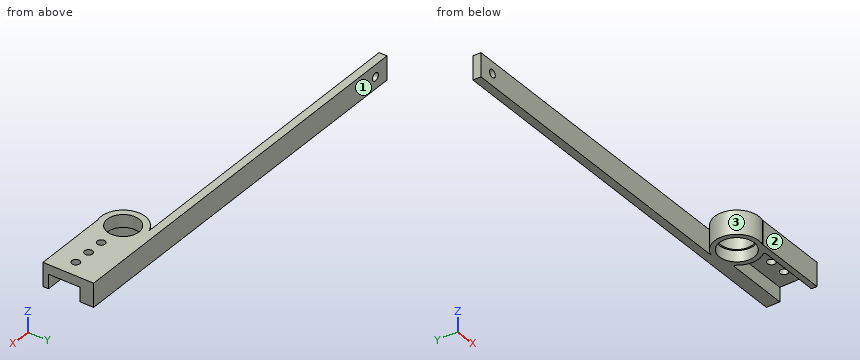
```python
from build123d import *

# Parameters (mm, degrees)
SKETCH_1_W          = 40
SKETCH_1_H          = 20
EXTRUDE_1_DEPTH     = 6
SKETCH_2_R          = 2.5
CUT_EXTRUDE_1_DEPTH = 24.151673806
EXTRUDE_START       = -15
EXTRUDE_2_OUTLINE_R = 11
EXTRUDE_2_DEPTH     = 15
EXTRUDE_START_2     = -8
SKETCH_5_R          = 11
SKETCH_5_R_2        = 10
EXTRUDE_3_DEPTH     = 8
SKETCH_8_W          = 15
SKETCH_8_H          = 5
EXTRUDE_4_DEPTH     = 500
SKETCH_9_W          = 4.037306924
SKETCH_9_H          = 3.364422437
EXTRUDE_5_DEPTH     = 15
SKETCH_11_W         = 261.320344598
SKETCH_11_H         = 37.265148186
CUT_EXTRUDE_2_DEPTH = 482.183177179
SKETCH_12_R         = 2.5
CUT_EXTRUDE_3_DEPTH = 237.730557242


# Read off the part's stored shape, not the designer's step: 凸台-拉伸2
with BuildPart() as part:
    # 草图1 → 凸台-拉伸1 (new body)
    with BuildSketch(Plane.XY):
        Rectangle(SKETCH_1_W, SKETCH_1_H)
    extrude(amount=EXTRUDE_1_DEPTH)

    # 草图2 → 切除-拉伸1 (cut, through all)
    with BuildSketch(Plane.XY.offset(6)):
        with Locations((10, 0)):
            Circle(SKETCH_2_R)
        with Locations((-1, 0)):
            Circle(SKETCH_2_R)
        with Locations((-12, 0)):
            Circle(SKETCH_2_R)
    extrude(amount=-CUT_EXTRUDE_1_DEPTH, mode=Mode.SUBTRACT)

    # 凸台-拉伸2 outline → 凸台-拉伸2 (add)
    with BuildSketch(Plane.XY.offset(6).offset(EXTRUDE_START)):
        with BuildLine():
            Line((20, 10), (20, 13.5))
            Line((20, 13.5), (-26.893967141, 13.5))
            Line((-26.893967141, 13.5), (-26.893967141, 13.384337644))
            ThreePointArc((-26.893967141, 13.384337644), (-45, 0), (-26.893967141, -13.384337644))
            Line((-26.893967141, -13.384337644), (-26.893967141, -13.5))
            Line((-26.893967141, -13.5), (20, -13.5))
            Line((20, -13.5), (20, -10))
            Line((20, -10), (-20, -10))
            Line((-20, -10), (-20, -8.660254038))
            ThreePointArc((-20, -8.660254038), (-17, 0), (-20, 8.660254038))
            Line((-20, 8.660254038), (-20, 10))
            Line((-20, 10), (20, 10))
        make_face()
        with Locations((-31, 0)):
            Circle(EXTRUDE_2_OUTLINE_R, mode=Mode.SUBTRACT)
    extrude(amount=EXTRUDE_2_DEPTH)

    # 草图5 → 凸台-拉伸3 (add)
    with BuildSketch(Plane.XY.offset(6).offset(EXTRUDE_START_2)):
        with Locations((-31, 0)):
            Circle(SKETCH_5_R)
        with Locations((-31, 0)):
            Circle(SKETCH_5_R_2, mode=Mode.SUBTRACT)
    extrude(amount=EXTRUDE_3_DEPTH)

    # 草图8 → 凸台-拉伸4 (add)
    with BuildSketch(Plane(origin=(20, 0, 0), x_dir=(0, 0, -1), z_dir=(1, 0, 0))):
        with Locations((1.5, 16)):
            Rectangle(SKETCH_8_W, SKETCH_8_H)
    extrude(amount=-EXTRUDE_4_DEPTH)

    # 草图9 → 凸台-拉伸5 (add, through all)
    with BuildSketch(Plane(origin=(0, 0, -9), x_dir=(-1, 0, 0), z_dir=(0, 0, -1))):
        with Locations((26.475334378, 14.151164675)):
            Rectangle(SKETCH_9_W, SKETCH_9_H)
    extrude(amount=-EXTRUDE_5_DEPTH)

    # 草图11 → 切除-拉伸2 (cut, through all)
    with BuildSketch(Plane(origin=(0, 18.5, 0), x_dir=(1, 0, 0), z_dir=(0, 1, 0))):
        with Locations((-364.976425965, 6.732710128)):
            Rectangle(SKETCH_11_W, SKETCH_11_H)
    extrude(amount=-CUT_EXTRUDE_2_DEPTH, mode=Mode.SUBTRACT)

    # 草图12 → 切除-拉伸3 (cut, through all)
    with BuildSketch(Plane(origin=(0, 18.5, 0), x_dir=(1, 0, 0), z_dir=(0, 1, 0))):
        with Locations(Location((-224.316253666, 1.5, 0), (0, 0, 270))):
            Circle(SKETCH_12_R)
    extrude(amount=-CUT_EXTRUDE_3_DEPTH, mode=Mode.SUBTRACT)


solid = part.part
```
For this review, take the finished solid that the model builds, in its own axes (mm). Face numbers are marked on the shaded views. Give positions to 0.01 mm unless a question says otherwise; leave off trailing zeros. Write each loop counter-clockwise with the first axis right and the second up, starting at its lowest first coordinate (ties: lowest second). Pieces come first, ordered by that corner, then holes.
Item 1: Take a section at D-D (y = 5). Give the boundary of the cut face in (x, z), and give its area (3 significant figures).
Item 2: Take a section at C-C (x = -146). Give the boundary of the cut face in (y, z).
Item 3: Take a section at A-A (x = -12). Give the boundary of the cut face in (y, z), and give its area (3 significant figures).
Item 4: The part is to be moulded in two halves that separate along Y. For the marked faces 1, 2 and 3, say which applies: +Y half, -Y half, draft (parallel to the pull), parting line (faces both ways), or undercut.
Item 5: Take a section at B-B (y = -5.5). Give the boundary of the cut face in (x, z).
Item 6: Insertion check: P1, Ø6.5, axis at x = 10, y = 0, coming from the -Z side; P2, Ø7.5, axis at x = -8.5, z = -2.5, coming from the -Y side; P3, Ø4, axis at x = -66, z = 0, coming from the -Y side. Each pin has a flat end and moves straight along its axis. Give the tip position at first contact, or say it passes through.
Item 7: Wall thickness on probe 1 along Y at (x, z) = (-31, -5.25); probe 2 along X at (y, z) = (-1, 1); probe 3 along Y at (x, z) = (-1, 4.3): over which ranges is each line inside the solid? List them lowest first.
Established:
1. outline: (-44.08, -9) - (-40.8, -9) - (-40.8, -2) - (-39.66, -2) - (-39.66, 6) - (-44.08, 6) - close; (-22.34, -2) - (-21.2, -2) - (-21.2, -9) - (-17.92, -9) - (-17.92, 0) - (20, 0) - (20, 6) - (-22.34, 6) - close
1. area: 344 mm2
2. outline: (13.5, -9) - (18.5, -9) - (18.5, 6) - (13.5, 6) - close
3. outline: (-13.5, -9) - (-10, -9) - (-10, 0) - (-2.5, 0) - (-2.5, 6) - (-13.5, 6) - close; (2.5, 0) - (10, 0) - (10, -9) - (18.5, -9) - (18.5, 6) - (2.5, 6) - close
3. area: 270 mm2
4. face 1: +Y half
4. face 2: -Y half
4. face 3: undercut
5. outline: (-43.87, -9) - (-40.53, -9) - (-40.53, -2) - (-39.35, -2) - (-39.35, 6) - (-43.87, 6) - close; (-22.65, -2) - (-21.47, -2) - (-21.47, -9) - (-18.13, -9) - (-18.13, 0) - (20, 0) - (20, 6) - (-22.65, 6) - close
6. P1: stops at z = 0
6. P2: stops at y = -13.5
6. P3: stops at y = 13.5
7. probe 1: y = -14 to -11, 11 to 18.5
7. probe 2: x = -44.96 to -40.95, -21.05 to -14.29, -9.71 to -3.29, 1.29 to 7.71, 12.29 to 20
7. probe 3: y = -13.5 to -2.5, 2.5 to 18.5
